from build123d import *

# Parameters (mm, degrees)
ESQUISSE1_R                              = 5.97
BOSS_EXTRU_1_DEPTH                       = 1.4
ESQUISSE2_R                              = 4.85
BOSS_EXTRU_2_DEPTH                       = 14.1
ESQUISSE3_R                              = 3.97
ESQUISSE3_R_2                            = 2.75
BOSS_EXTRU_3_DEPTH                       = 8.26
ESQUISSE4_R                              = 1
BOSS_EXTRU_4_DEPTH                       = 5
ENL_V_MAT_EXTRU_1_REACH                  = 18.434
ENL_V_MAT_EXTRU_1_END_RADIUS             = 3.97
ESQUISSE5_W                              = 8.26
ESQUISSE5_H                              = 0.57
ENL_V_MAT_EXTRU_1_DIRECTION_2_REACH      = 18.434
ENL_V_MAT_EXTRU_1_DIRECTION_2_END_RADIUS = 3.97
ESQUISSE6_R                              = 3.62
ESQUISSE6_W                              = 0.51
ESQUISSE6_H                              = 3
BOSS_EXTRU_5_DEPTH                       = 5.2
ESQUISSE7_W                              = 0.51
ESQUISSE7_H                              = 3
BOSS_EXTRU_6_DEPTH                       = 7.4


with BuildPart() as part:
    # Esquisse1 → Boss.-Extru.1 (new body)
    with BuildSketch(Plane.XY):
        Circle(ESQUISSE1_R)
    extrude(amount=BOSS_EXTRU_1_DEPTH)

    # Esquisse2 → Boss.-Extru.2 (add)
    with BuildSketch(Plane(origin=(0, 0, 0), x_dir=(-1, 0, 0), z_dir=(0, 0, -1))):
        Circle(ESQUISSE2_R)
    extrude(amount=BOSS_EXTRU_2_DEPTH)

    # Esquisse3 → Boss.-Extru.3 (add)
    with BuildSketch(Plane.XY.offset(1.4)):
        Circle(ESQUISSE3_R)
        Circle(ESQUISSE3_R_2, mode=Mode.SUBTRACT)
    extrude(amount=BOSS_EXTRU_3_DEPTH)

    # Esquisse4 → Boss.-Extru.4 (add)
    with BuildSketch(Plane.XY.offset(1.4)):
        Circle(ESQUISSE4_R)
    extrude(amount=BOSS_EXTRU_4_DEPTH)

    # Enlèv. mat.-Extru.1: up to this cylinder (the profile starts inside it)
    enl_v_mat_extru_1_end = Plane(origin=(0, 0, 5.53), z_dir=(0, 0, -1)) * Cylinder(ENL_V_MAT_EXTRU_1_END_RADIUS, 45.808, mode=Mode.PRIVATE)
    # Esquisse5 → Enlèv. mat.-Extru.1 (cut, up to the surface)
    with BuildSketch(Plane(origin=(0, 0, 0), x_dir=(0, 0, -1), z_dir=(1, 0, 0)), mode=Mode.PRIVATE) as enl_v_mat_extru_1_sk1:
        with Locations((-5.53, 3.685)):
            Rectangle(ESQUISSE5_W, ESQUISSE5_H)
    enl_v_mat_extru_1_tool1 = extrude(enl_v_mat_extru_1_sk1.sketch, amount=-ENL_V_MAT_EXTRU_1_REACH, mode=Mode.PRIVATE) & enl_v_mat_extru_1_end
    add(enl_v_mat_extru_1_tool1.solids().sort_by_distance((0, 3.685, 5.53))[0], mode=Mode.SUBTRACT)

    # Enlèv. mat.-Extru.1 direction 2: up to this cylinder (the profile starts inside it)
    enl_v_mat_extru_1_direction_2_end = Plane(origin=(0, 0, 5.53), z_dir=(0, 0, -1)) * Cylinder(ENL_V_MAT_EXTRU_1_DIRECTION_2_END_RADIUS, 45.808, mode=Mode.PRIVATE)
    # Esquisse5 → Enlèv. mat.-Extru.1 direction 2 (cut, up to the surface)
    with BuildSketch(Plane(origin=(0, 0, 0), x_dir=(0, 0, -1), z_dir=(1, 0, 0)), mode=Mode.PRIVATE) as enl_v_mat_extru_1_direction_2_sk1:
        with Locations((-5.53, 3.685)):
            Rectangle(ESQUISSE5_W, ESQUISSE5_H)
    enl_v_mat_extru_1_direction_2_tool1 = extrude(enl_v_mat_extru_1_direction_2_sk1.sketch, amount=ENL_V_MAT_EXTRU_1_DIRECTION_2_REACH, mode=Mode.PRIVATE) & enl_v_mat_extru_1_direction_2_end
    add(enl_v_mat_extru_1_direction_2_tool1.solids().sort_by_distance((0, 3.685, 5.53))[0], mode=Mode.SUBTRACT)

    # Esquisse6 → Boss.-Extru.5 (add)
    with BuildSketch(Plane(origin=(0, 0, -14.1), x_dir=(-1, 0, 0), z_dir=(0, 0, -1))):
        Circle(ESQUISSE6_R)
        with Locations((-4.595, 0)):
            Rectangle(ESQUISSE6_W, ESQUISSE6_H)
    extrude(amount=BOSS_EXTRU_5_DEPTH)

    # Esquisse7 → Boss.-Extru.6 (add)
    with BuildSketch(Plane(origin=(0, 0, -19.3), x_dir=(-1, 0, 0), z_dir=(0, 0, -1))):
        with Locations((3.365, 0)):
            Rectangle(ESQUISSE7_W, ESQUISSE7_H)
    extrude(amount=BOSS_EXTRU_6_DEPTH)


solid = part.part
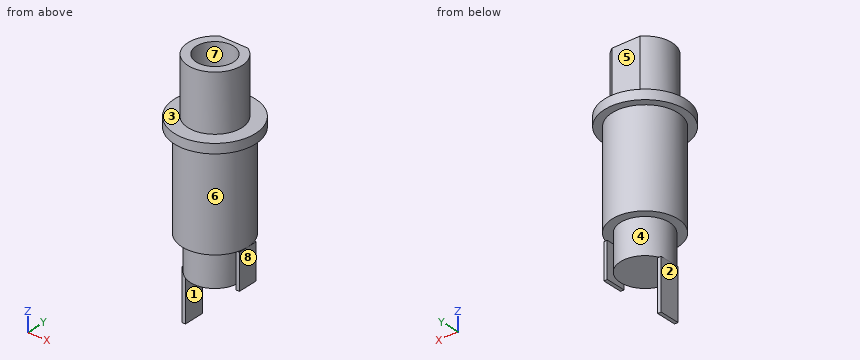
Here's how the part is built. I have some questions about the finished solid (model axes, mm). Face numbers are marked on the shaded views. A direction names the side the tool comes from. Round coordinates to 2 decimals unless told otherwise and drop trailing zeros. Loops run counter-clockwise (first coordinate to the right, second up) from the corner with the lowest first, then second, coordinate; pieces in that order, holes last. Notation, with made-up numbers: M 26,1.5 L 60,1.5 A5 ccw 60,10.5 Z; hole C -14.5,26.25 d1. An arc over 180 degrees is marked long. Write each question's results on one line, items separated by ' | '. Start each with the question number.
(1) I want a section at D-D (y = -3.25). Please give me the cut outline in (x, z).
(2) I want a section at A-A (x = 0). Please give me the cut outline in (y, z).
(3) Will these pins go through, and if not, where does the flat tip stop? P1, Ø0.6, axis at x = 4.5, z = -18, coming from the +Y side; P2, Ø5, axis at x = 1, z = -22, coming from the +Y side; P3, Ø1.5, axis at x = 4.5, y = -3, coming from the -Z side; P4, Ø1.5, axis at y = -0.5, z = -22.5, coming from the +X side.
(4) Thinking about a two-plate mould opening in Y: for the marked faces 5, 6, 7 and 8, which applies, pulls with the +Y half, pulls with the -Y half, needs draft (parallel to the pull), parting line crosses it, or undercut?
(5) On a 3-axis mill with a long thin cutter (end or side, diameter ignored), from which of +Z, -Z, +X, -X, +Y, -Y can I reach the whole of each face in a straight line? I mean the marked faces 1, 2, 3 and 4. Say none if no direction works.
(6) I want a section at B-B (z = -15). Please give me the cut outline in (x, y), then the cut area to 3 significant figures.
(7) If I drill on probe 1 along Y at (x, z) = (0, 4.5); probe 2 along Y at (x, z) = (0, 6.5); probe 3 along Z at (x, y) = (-2.75, 5), over which ranges is the centre line in solid material (lowest first)? Write a range as from..to.
(8) I want a section at C-C (z = 3). Please give me the cut outline in (x, y), then the cut area to 3 significant figures.
Solved:
1) outline: M -5.01,0 L -3.6,0 L -3.6,-14.1 L -1.59,-14.1 L -1.59,-19.3 L 1.59,-19.3 L 1.59,-14.1 L 3.6,-14.1 L 3.6,0 L 5.01,0 L 5.01,1.4 L 2.28,1.4 L 2.28,9.66 L -2.28,9.66 L -2.28,1.4 L -5.01,1.4 Z
2) outline: M -5.97,0 L -4.85,0 L -4.85,-14.1 L -3.62,-14.1 L -3.62,-19.3 L 3.62,-19.3 L 3.62,-14.1 L 4.85,-14.1 L 4.85,0 L 5.97,0 L 5.97,1.4 L 3.4,1.4 L 3.4,9.66 L 2.75,9.66 L 2.75,1.4 L 1,1.4 L 1,6.4 L -1,6.4 L -1,1.4 L -2.75,1.4 L -2.75,9.66 L -3.97,9.66 L -3.97,1.4 L -5.97,1.4 Z
3) P1: stops at y = 1.5 | P2: passes through | P3: stops at z = -14.1 | P4: stops at x = -3.11
4) face 5: pulls with the +Y half | face 6: parting line crosses it | face 7: undercut | face 8: needs draft
5) face 1: -Z, +X, +Y, -Y | face 2: -Z, -X, +Y, -Y | face 3: +Z | face 4: none
6) outline: C 0,0 d7.24; M 4.34,-1.5 L 4.85,-1.5 L 4.85,1.5 L 4.34,1.5 Z | area: 42.7 mm²
7) probe 1: y = -3.97..-2.75, -1..1, 2.75..3.4 | probe 2: y = -3.97..-2.75, 2.75..3.4 | probe 3: z = 0..1.4
8) outline: M -2.05,3.4 A3.97 ccw long 2.05,3.4 Z; C 0,0 d2; hole C 0,0 d5.5 | area: 27.3 mm²
